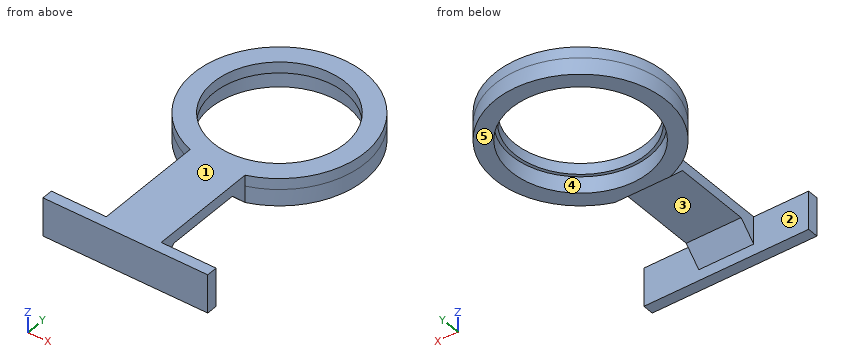
```python
from build123d import *

# Parameters (mm, degrees)
BOSS_EXTRUDE1_DEPTH      = 2
BOSS_EXTRUDE1_DEPTH_BACK = 1
SKETCH1_R                = 12.575
SKETCH2_R                = 12
BOSS_EXTRUDE2_DEPTH      = 2
CUT_EXTRUDE1_DEPTH       = 43.30766223
BOSS_EXTRUDE3_DEPTH      = 2


with BuildPart() as part:
    # Sketch1 → Boss-Extrude1 (new, two sides: drawn at the far end of the back side and taken through both)
    with BuildSketch(Plane.XY.offset(-BOSS_EXTRUDE1_DEPTH_BACK)):
        with BuildLine():
            Line((5, -34.750614394), (15, -34.750614394))
            Line((15, -34.750614394), (15, -36.750614394))
            Line((15, -36.750614394), (-15, -36.750614394))
            Line((-15, -36.750614394), (-15, -34.750614394))
            Line((-15, -34.750614394), (-5, -34.750614394))
            Line((-5, -34.750614394), (-5, -14.750614394))
            ThreePointArc((-5, -14.750614394), (0, 15.575), (5, -14.750614394))
            Line((5, -14.750614394), (5, -34.750614394))
        make_face()
        Circle(SKETCH1_R, mode=Mode.SUBTRACT)
    extrude(amount=BOSS_EXTRUDE1_DEPTH + BOSS_EXTRUDE1_DEPTH_BACK)

    # Sketch2 → Boss-Extrude2 (add)
    with BuildSketch(Plane.XY.offset(2)):
        with BuildLine():
            Line((-5, -14.750614394), (-5, -34.750614394))
            Line((-5, -34.750614394), (-15, -34.750614394))
            Line((-15, -34.750614394), (-15, -36.750614394))
            Line((-15, -36.750614394), (15, -36.750614394))
            Line((15, -36.750614394), (15, -34.750614394))
            Line((15, -34.750614394), (5, -34.750614394))
            Line((5, -34.750614394), (5, -14.750614394))
            ThreePointArc((5, -14.750614394), (0, 15.575), (-5, -14.750614394))
        make_face()
        Circle(SKETCH2_R, mode=Mode.SUBTRACT)
    extrude(amount=BOSS_EXTRUDE2_DEPTH)

    # Sketch4 → Cut-Extrude1 (cut, through all)
    with BuildSketch(Plane.ZY.offset(5)):
        Polygon((-1, -14.750614394), (2, -17.750614394), (2, -31.750614394), (-1, -34.750614394), align=None)
    extrude(amount=-CUT_EXTRUDE1_DEPTH, mode=Mode.SUBTRACT)

    # Sketch5 → Boss-Extrude3 (add)
    with BuildSketch(Plane(origin=(0, 0, -1), x_dir=(-1, 0, 0), z_dir=(0, 0, -1))):
        Polygon((15, -34.750614394), (5, -34.750614394), (-5, -34.750614394), (-15, -34.750614394), (-15, -36.750614394), (15, -36.750614394), align=None)
    extrude(amount=BOSS_EXTRUDE3_DEPTH)


solid = part.part
```
Design review of the part built by this model. Coordinates are the model's own, in mm. Face numbers are marked on the shaded views. A direction names the side the tool comes from. Give positions to 0.01 mm unless a question says otherwise; leave off trailing zeros. Loops run counter-clockwise (first coordinate to the right, second up) from the corner with the lowest first, then second, coordinate; pieces in that order, holes last. Notation, with made-up numbers: M 2,16.25 L 29,16.25 A25 ccw 29,54.25 Z; hole C 39.5,60 d8. An arc over 180 degrees is marked long. Return JSON: item names as keys, results as strings. Group by question number.
Item 1: We need section C-C (z = 1). Give the boundary of the cut face in (x, y) (3 decimals), and give its area (3 significant figures).
Item 2: We need section B-B (y = 0). Give the boundary of the cut face in (x, z) (3 decimals).
Item 3: Tool access review of the marked faces 1, 2 and 3: name each direction out of +Z, -Z, +X, -X, +Y, -Y from which nothing blocks a thin tool from reaching the whole face with its end or side.
Item 4: Mouldability with a two-part tool opening along X and no side actions: class the marked faces 4 and 5 as released by +X, released by -X, zero draft, split by the parting line, or undercut.
Item 5: We need section D-D (x = 6.5). Give the boundary of the cut face in (y, z), and give its area (3 significant figures).
Item 6: For probe 1 along Y at (x, z) = (0, 3.3) (3 decimals); probe 2 along Y at (x, z) = (6.5, 1.25); probe 3 along Y at (x, z) = (8, 3.5), list the stretches that pass through material, from the lowest coordinate up.
Item 7: We need section A-A (x = 0). Give the boundary of the cut face in (y, z) (3 decimals).
Item 8: Insertion check: pin 1 Ø4 at (y, z) = (-28, 2) entering from -X; pin 2 Ø1.5 at (y, z) = (-28, 2) entering from +X; pin 3 Ø1.5 at (y, z) = (-6.5, -2) entering from +X; pin 4 Ø1 at (x, z) = (-7, -1) entering from +Y. Each pin has a flat end and moves straight along its axis. Give the tip position at first contact, or say it passes through.
Output:
{
 "1": {"outline": "M -15,-36.751 L 15,-36.751 L 15,-34.751 L 5,-34.751 L 5,-32.751 L -5,-32.751 L -5,-34.751 L -15,-34.751 Z; M -5,-16.751 L 5,-16.751 L 5,-14.751 A15.575 ccw long -5,-14.751 Z; hole C 0,0 d25.15", "area": "360 mm^2"},
 "2": {"outline": "M -15.575,-1 L -12.575,-1 L -12.575,2 L -12,2 L -12,4 L -15.575,4 Z; M 12,2 L 12.575,2 L 12.575,-1 L 15.575,-1 L 15.575,4 L 12,4 Z"},
 "3": {"face 1": "+Z, +X, -X, +Y, -Y", "face 2": "-Z", "face 3": "-Z, +X, -X"},
 "4": {"face 4": "undercut", "face 5": "zero draft"},
 "5": {"outline": "M -36.75,-3 L -34.75,-3 L -34.75,4 L -36.75,4 Z; M -14.15,-1 L -10.76,-1 L -10.76,2 L -10.09,2 L -10.09,4 L -14.15,4 Z; M 10.09,2 L 10.76,2 L 10.76,-1 L 14.15,-1 L 14.15,4 L 10.09,4 Z", "area": "50.6 mm^2"},
 "6": {"probe 1": "y = -36.751 to -12, 12 to 15.575", "probe 2": "y = -36.75 to -34.75, -14.15 to -10.76, 10.76 to 14.15", "probe 3": "y = -36.75 to -34.75, -13.36 to -8.94, 8.94 to 13.36"},
 "7": {"outline": "M -36.751,-3 L -34.751,-3 L -34.751,-1 L -31.751,2 L -17.751,2 L -14.751,-1 L -12.575,-1 L -12.575,2 L -12,2 L -12,4 L -36.751,4 Z; M 12,2 L 12.575,2 L 12.575,-1 L 15.575,-1 L 15.575,4 L 12,4 Z"},
 "8": {"pin 1": "stops at x = -5", "pin 2": "stops at x = 5", "pin 3": "passes through", "pin 4": "stops at y = 14.15"}
}
